from build123d import *

# Parameters (mm, degrees)
BOSS_EXTRUDE1_DEPTH     = 20
FILLET1_R               = 5
CUT_EXTRUDE1_DEPTH      = 72.877952398
CUT_EXTRUDE1_DEPTH_BACK = 72.877952398
SKETCH2_R               = 2.2
SKETCH3_R               = 3.7
CUT_EXTRUDE2_DEPTH      = 8.846664929
CHAMFER2_SIZE           = 1
BOSS_EXTRUDE2_START     = -3.375
BOSS_EXTRUDE2_DEPTH     = 12.971664929
BOSS_EXTRUDE3_DEPTH     = 13.153335071
SKETCH6_R               = 3
CUT_EXTRUDE3_DEPTH      = 6.2
CUT_EXTRUDE4_DEPTH      = 74.770702766
CUT_EXTRUDE4_DEPTH_BACK = 74.770702766
SKETCH7_R               = 2.2


with BuildPart() as part:
    # Sketch1 → Boss-Extrude1 (new body)
    with BuildSketch(Plane(origin=(-19.912110777, 0, 0), x_dir=(0, 0, -1), z_dir=(1, 0, 0))):
        with BuildLine():
            Line((-52.5, 12.196664929), (-44.846664929, 12.196664929))
            ThreePointArc((-44.846664929, 12.196664929), (-32.5, 24.543329858), (-20.153335071, 12.196664929))
            Line((-20.153335071, 12.196664929), (-7.5, 12.196664929))
            Line((-7.5, 12.196664929), (-7.5, 28.543329858))
            Line((-7.5, 28.543329858), (-57.5, 28.543329858))
            Line((-57.5, 28.543329858), (-57.5, 12.196664929))
            Line((-57.5, 12.196664929), (-52.5, 12.196664929))
        make_face()
    extrude(amount=-BOSS_EXTRUDE1_DEPTH)

    # Fillet1
    fillet1_edges = [part.edges().sort_by_distance(p)[0] for p in [
        (-39.912110777, 20.369997393, 7.5),
        (-39.912110777, 20.369997393, 57.5),
        (-19.912110777, 20.369997393, 57.5),
        (-19.912110777, 20.369997393, 7.5),
    ]]
    fillet(fillet1_edges, radius=FILLET1_R)

    # Sketch2 → Cut-Extrude1 (cut, two sides: drawn at the far end of the back side and taken through both)
    with BuildSketch(Plane(origin=(0, 28.543329858, 0), x_dir=(1, 0, 0), z_dir=(0, 1, 0)).offset(-CUT_EXTRUDE1_DEPTH_BACK)):
        with Locations(Location((-29.912110777, -51.172876859, 0), (0, 0, 270))):
            Circle(SKETCH2_R)
        with Locations(Location((-29.912110777, -13.827123141, 0), (0, 0, 270))):
            Circle(SKETCH2_R)
    extrude(amount=CUT_EXTRUDE1_DEPTH + CUT_EXTRUDE1_DEPTH_BACK, mode=Mode.SUBTRACT)

    # Sketch3 → Cut-Extrude2 (cut)
    with BuildSketch(Plane(origin=(0, 28.543329858, 0), x_dir=(1, 0, 0), z_dir=(0, 1, 0))):
        with Locations(Location((-29.912110777, -51.172876859, 0), (0, 0, 270))):
            Circle(SKETCH3_R)
        with Locations(Location((-29.912110777, -13.827123141, 0), (0, 0, 270))):
            Circle(SKETCH3_R)
    extrude(amount=-CUT_EXTRUDE2_DEPTH, mode=Mode.SUBTRACT)

    # Chamfer2
    chamfer2_edges = [part.edges().sort_by_distance(p)[0] for p in [
        (-29.912110777, 28.543329858, 47.472876859),
        (-29.912110777, 28.543329858, 10.127123141),
    ]]
    chamfer(chamfer2_edges, length=CHAMFER2_SIZE)

    # Sketch4 → Boss-Extrude2 (add)
    with BuildSketch(Plane(origin=(0, 28.543329858, 0), x_dir=(1, 0, 0), z_dir=(0, 1, 0)).offset(BOSS_EXTRUDE2_START)):
        with BuildLine():
            Line((-0.4, -47.5), (-19.912110777, -47.5))
            Line((-19.912110777, -47.5), (-19.912110777, -52.5))
            ThreePointArc((-19.912110777, -52.5), (-21.376576871, -56.035533906), (-24.912110777, -57.5))
            Line((-24.912110777, -57.5), (-0.4, -57.5))
            Line((-0.4, -57.5), (-0.4, -47.5))
        make_face()
        with BuildLine():
            Line((-19.912110777, -0.4), (-24.912110777, -0.4))
            Line((-24.912110777, -0.4), (-24.912110777, -7.5))
            ThreePointArc((-24.912110777, -7.5), (-21.376576871, -8.964466094), (-19.912110777, -12.5))
            Line((-19.912110777, -12.5), (-19.912110777, -0.4))
        make_face()
    extrude(amount=-BOSS_EXTRUDE2_DEPTH)

    # Sketch5 → Boss-Extrude3 (add)
    with BuildSketch(Plane(origin=(0, 28.543329858, 0), x_dir=(1, 0, 0), z_dir=(0, 1, 0))):
        with BuildLine():
            Line((-29.912110777, -46.472876859), (-24.38878903, -46.472876859))
            Line((-24.38878903, -46.472876859), (-24.38878903, -18.527123141))
            Line((-24.38878903, -18.527123141), (-29.912110777, -18.527123141))
            ThreePointArc((-29.912110777, -18.527123141), (-32.964467867, -17.401072804), (-34.554225923, -14.562491734))
            Line((-34.554225923, -14.562491734), (-39.912110777, -14.562491734))
            Line((-39.912110777, -14.562491734), (-39.912110777, -50.437508266))
            Line((-39.912110777, -50.437508266), (-34.554225923, -50.437508266))
            ThreePointArc((-34.554225923, -50.437508266), (-32.964467867, -47.598927196), (-29.912110777, -46.472876859))
        make_face()
    extrude(amount=BOSS_EXTRUDE3_DEPTH)

    # Sketch6 → Cut-Extrude3 (cut)
    with BuildSketch(Plane(origin=(0, 41.696664929, 0), x_dir=(1, 0, 0), z_dir=(0, 1, 0))):
        with Locations(Location((-32.150449903, -32.5, 0), (0, 0, 270))):
            Circle(SKETCH6_R)
    extrude(amount=-CUT_EXTRUDE3_DEPTH, mode=Mode.SUBTRACT)

    # Sketch7 → Cut-Extrude4 (cut, two sides: drawn at the far end of the back side and taken through both)
    with BuildSketch(Plane(origin=(0, 35.496664929, 0), x_dir=(1, 0, 0), z_dir=(0, 1, 0)).offset(-CUT_EXTRUDE4_DEPTH_BACK)):
        with Locations(Location((-32.150449903, -32.5, 0), (0, 0, 270))):
            Circle(SKETCH7_R)
    extrude(amount=CUT_EXTRUDE4_DEPTH + CUT_EXTRUDE4_DEPTH_BACK, mode=Mode.SUBTRACT)


solid = part.part
Could you check a few things on this model? Use its own coordinates, in mm. A direction names the side the tool comes from. Give positions to 0.01 mm unless a question says otherwise; leave off trailing zeros. Order: outer loops, then holes, each group sorted by start corner. A loop starts at its lowest first (then second) coordinate and runs counter-clockwise, first axis right, second up. Notation, with made-up numbers: (6.25, -34) - (12.25, -34) arc R29 cw to (12.25, -7) - close; hole circle Ø6 at (64, 72). An arc over 180 degrees is marked (long way). One line per item, written item: value. Start each with the question number.
1. Imagine slicing it at D-D on x = -14. List the corners of the cut face in (y, z) for me.
2. Thinking about a two-plate mould opening in X: for faces 1 (the face through (-32.93, 35.03, 17.43)), 2 (the face through (-27.73, 15.89, 13.54)), 3 (the face through (-24, 28.543, 32)), which applies, +X half, -X half, draft (parallel to the pull), parting line (faces both ways), or undercut?
3. Imagine slicing it at C-C on z = 21. List the corners of the cut face in (x, y) for me, plus the area to 3 significant figures.
4. Imagine slicing it at B-B on y = 31.75. List the corners of the cut face in (x, z) for me, plus the area to 3 significant figures.
5. For faces 4 (the face through (-37, 35, 14.562)), 5 (the face through (-10, 19, 47.5)), 6 (the face through (-30, 35.497, 34)), which set-ups out of +Z, -Z, +X, -X, +Y, -Y let a thin tool reach every point of the face, with its end or its side?
6. Imagine slicing it at A-A on z = 32.5. List the corners of the cut face in (x, y) for me.
7. If I drill on probe 1 along X at (y, z) = (31, 32.5); probe 2 along X at (y, z) = (37.75, 32.5); probe 3 along X at (y, z) = (25.75, 37.5), over which ranges is the centre line in solid material (lowest first)?
8. For P1, Ø3, axis at x = -29, y = 22, coming from the -Z side; P2, Ø4, axis at x = -23.5, z = 4, coming from the +Y side; P3, Ø5, axis at y = 18.5, z = 17.5, coming from the +X side, each with a flat end and sliding along its axis, tell me the tip position at first contact or that it passes through.
Values:
1. outline: (12.2, 47.5) - (25.17, 47.5) - (25.17, 57.5) - (12.2, 57.5) - close
2. face 1: +X half
2. face 2: undercut
2. face 3: draft
3. outline: (-39.91, 16.69) - (-19.91, 16.69) - (-19.91, 28.54) - (-24.39, 28.54) - (-24.39, 41.7) - (-39.91, 41.7) - close
3. area: 441 mm²
4. outline: (-39.91, 14.56) - (-34.55, 14.56) arc R4.7 cw to (-29.91, 18.53) - (-24.39, 18.53) - (-24.39, 46.47) - (-29.91, 46.47) arc R4.7 cw to (-34.55, 50.44) - (-39.91, 50.44) - close; hole circle Ø4.4 at (-32.15, 32.5)
4. area: 470 mm²
5. face 4: -Z, +X, -X, +Y
5. face 5: -Z, +X, +Y, -Y
5. face 6: +Y
6. outline: (-39.91, 24.54) - (-34.35, 24.54) - (-34.35, 35.5) - (-35.15, 35.5) - (-35.15, 41.7) - (-39.91, 41.7) - close; (-29.95, 24.54) - (-19.91, 24.54) - (-19.91, 28.54) - (-24.39, 28.54) - (-24.39, 41.7) - (-29.15, 41.7) - (-29.15, 35.5) - (-29.95, 35.5) - close
7. probe 1: -39.91 to -34.35, -29.95 to -24.39
7. probe 2: -39.91 to -35.15, -29.15 to -24.39
7. probe 3: -39.91 to -19.91
8. P1: z = 7.5
8. P2: y = 25.17
8. P3: x = -19.91
